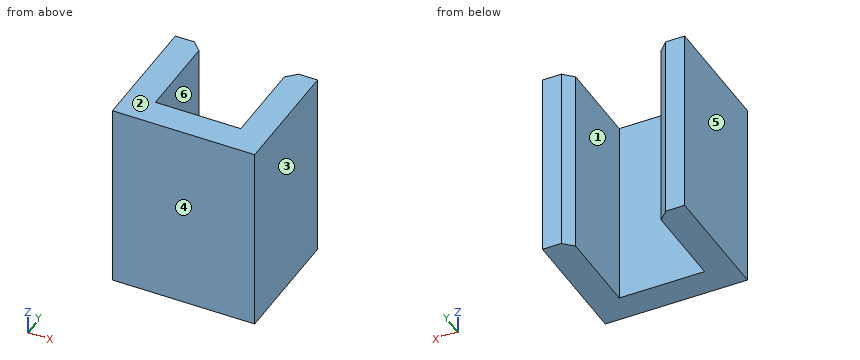
```python
from build123d import *

# Parameters (mm, degrees)
PAD_DEPTH    = 20
CHAMFER_SIZE = 1


with BuildPart() as part:
    # Sketch → Pad (new body)
    with BuildSketch(Plane.XY):
        Polygon((-7.5, 5), (-7.5, -8), (7.5, -8), (7.5, 5), (4.5, 5), (4.5, -5), (-4.5, -5), (-4.5, 5), align=None)
    extrude(amount=PAD_DEPTH)

    # Chamfer
    chamfer_edges = [part.edges().sort_by_distance(p)[0] for p in [
        (-4.5, 5, 10),
        (4.5, 5, 10),
    ]]
    chamfer(chamfer_edges, length=CHAMFER_SIZE)


solid = part.part
```
Here's how the part is built. I have some questions about the finished solid (model axes, mm). Face numbers are marked on the shaded views. A direction names the side the tool comes from. Coordinates: 2 decimals unless noted, no trailing zeros. Order: outer loops, then holes, each group sorted by start corner. A loop starts at its lowest first (then second) coordinate and runs counter-clockwise, first axis right, second up. Notation, with made-up numbers: (80, 57.5) - (134, 57.5) arc R17 cw to (134, 65.5) - close; hole circle Ø11 at (75.5, 53). An arc over 180 degrees is marked (long way). One line per question, with ' | ' between items.
(1) For the marked faces 1 and 2, which set-ups out of +Z, -Z, +X, -X, +Y, -Y let a thin tool reach every point of the face, with its end or its side?
Report:
face 1: +Z, -Z, +Y | face 2: +Z, +X, -X, +Y, -Y
(2) If we mould it in two halves opening along X, with no side actions, what happens to the marked faces 3, 4, 5 and 6? For each: pulls with the +X half, pulls with the -X half, needs draft (parallel to the pull), parting line crosses it, or undercut.
Report:
face 3: pulls with the +X half | face 4: needs draft | face 5: pulls with the -X half | face 6: undercut
(3) Suppose I cut it at D-D on x = -5. List the corners of the cut face in (y, z) for me, and give its area (3 significant figures).
Report:
outline: (-8, 0) - (4.5, 0) - (4.5, 20) - (-8, 20) - close | area: 250 mm2
(4) Suppose I cut it at B-B on z = 4.75. List the corners of the cut face in (x, y) for me.
Report:
outline: (-7.5, -8) - (7.5, -8) - (7.5, 5) - (5.5, 5) - (4.5, 4) - (4.5, -5) - (-4.5, -5) - (-4.5, 4) - (-5.5, 5) - (-7.5, 5) - close
(5) Suppose I cut it at A-A on y = -0.5. List the corners of the cut face in (x, z) for me.
Report:
outline: (-7.5, 0) - (-4.5, 0) - (-4.5, 20) - (-7.5, 20) - close; (4.5, 0) - (7.5, 0) - (7.5, 20) - (4.5, 20) - close
(6) If I drill on L1, parallel to X at y = -3.25, z = 14.75; L2, parallel to Y at x = 1.25, z = 15, over which ranges is the centre line in solid material (lowest first)?
Report:
L1: x = -7.5 to -4.5, 4.5 to 7.5 | L2: y = -8 to -5
(7) Suppose I cut it at C-C on x = 1.75. List the corners of the cut face in (y, z) for me.
Report:
outline: (-8, 0) - (-5, 0) - (-5, 20) - (-8, 20) - close
